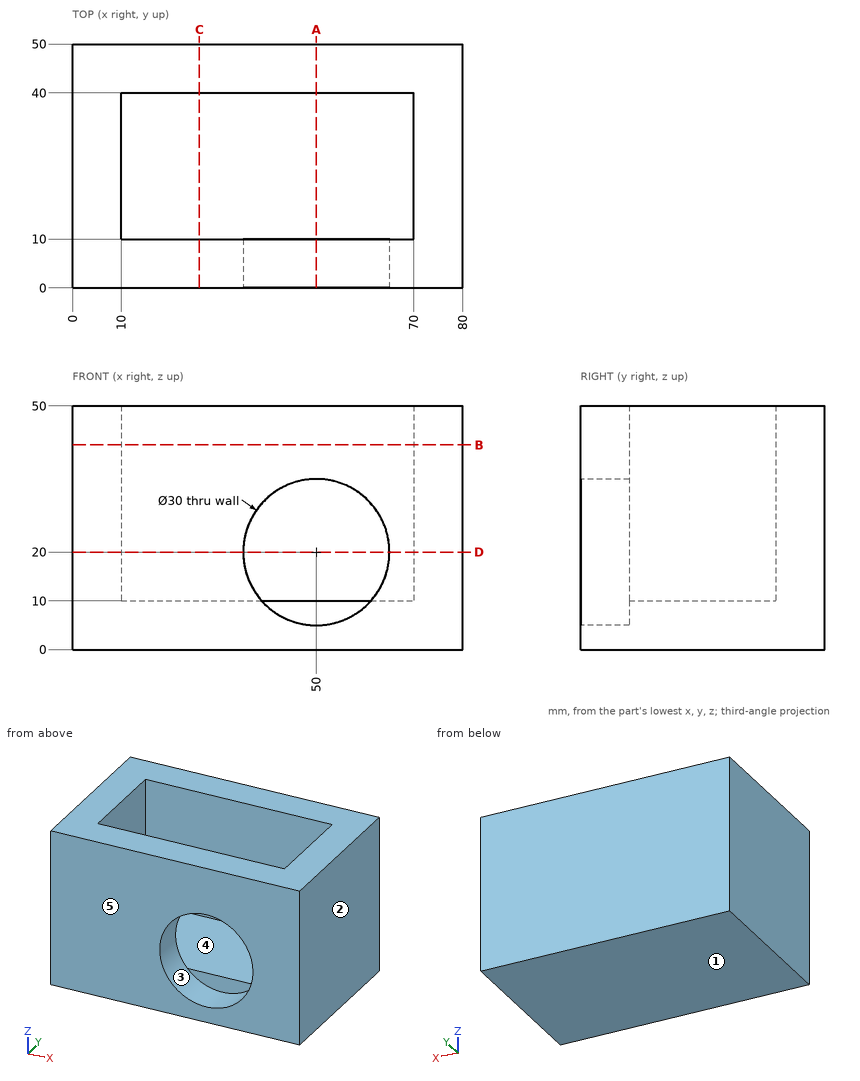
Can you work these out from the drawing? Everything is in mm from the part's minimum corner. A direction names the side the tool comes from. Give positions to 0.01 mm unless a question says otherwise; leave off trailing zeros. Order: outer loops, then holes, each group sorted by start corner. A loop starts at its lowest first (then second) coordinate and runs counter-clockwise, first axis right, second up.
Item 1: If we section it at A-A, the plane x = 50: Write out the boundary of the cut face in (y, z), plus the area to 3 significant figures.
Item 2: If we mould it in two halves opening along X, with no side actions, what happens to the marked faces 1, 2 and 3? For each: pulls with the +X half, pulls with the -X half, needs draft (parallel to the pull), parting line crosses it, or undercut.
Item 3: I'm going to push flat-ended pins straight in: pin 1 (3 mm diameter, centred on x = 47.5, y = 28, fed in from -Z); pin 2 (4 mm diameter, centred on x = 28.5, y = 25.5, fed in from +Z); pin 3 (1.5 mm diameter, centred on x = 51.5, z = 7, fed in from -Y). Where does each tip first touch, or does it pass through?
Item 4: For the marked faces 4 and 5, which set-ups out of +Z, -Z, +X, -X, +Y, -Y let a thin tool reach every point of the face, with its end or its side?
Item 5: If we section it at C-C, the plane x = 26: Write out the boundary of the cut face in (y, z).
Item 6: I need wall thicknesses on line 1 (X direction, y = 33.5, z = 41); line 2 (Z direction, x = 50, y = 6); line 3 (Y direction, x = 50, z = 39). Which ranges of each line are inside material? Lowest first, please.
Item 7: If we section it at B-B, the plane z = 42: Write out the boundary of the cut face in (x, y).
Item 8: If we section it at D-D, the plane z = 20: Write out the boundary of the cut face in (x, y).
Values:
1. outline: (0, 0) - (50, 0) - (50, 50) - (40, 50) - (40, 10) - (10, 10) - (10, 5) - (0, 5) - close; (0, 35) - (10, 35) - (10, 50) - (0, 50) - close
1. area: 1,000 mm2
2. face 1: needs draft
2. face 2: pulls with the +X half
2. face 3: undercut
3. pin 1: stops at z = 0
3. pin 2: stops at z = 10
3. pin 3: stops at y = 10
4. face 4: +Z
4. face 5: +Z, -Z, +X, -X, -Y
5. outline: (0, 0) - (50, 0) - (50, 50) - (40, 50) - (40, 10) - (10, 10) - (10, 50) - (0, 50) - close
6. line 1: x = 0 to 10, 70 to 80
6. line 2: z = 0 to 5, 35 to 50
6. line 3: y = 0 to 10, 40 to 50
7. outline: (0, 0) - (80, 0) - (80, 50) - (0, 50) - close; hole (10, 10) - (70, 10) - (70, 40) - (10, 40) - close
8. outline: (0, 0) - (35, 0) - (35, 10) - (10, 10) - (10, 40) - (70, 40) - (70, 10) - (65, 10) - (65, 0) - (80, 0) - (80, 50) - (0, 50) - close
